Read the model definition and answer for the solid it produces. Units are mm, in the model's axes. Coordinates: 2 decimals unless noted, no trailing zeros. Loops run counter-clockwise (first coordinate to the right, second up) from the corner with the lowest first, then second, coordinate; pieces in that order, holes last. Notation, with made-up numbers: (68, -16.75) -> (76, -16.75) arc R23 ccw to (76, 14.25) -> close; hole circle Ø6 at (-24.5, 16.25). An arc over 180 degrees is marked (long way). Answer in a Markdown table with one row per item.
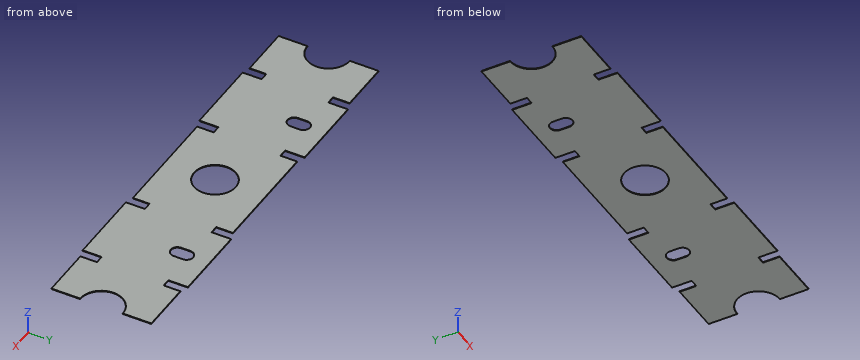
```python
from build123d import *

# Parameters (mm, degrees)
SKETCH_1_R      = 5
EXTRUDE_1_DEPTH = 0.15


with BuildPart() as part:
    # Эскиз1 → Бобышка-Вытянуть1 (new body)
    with BuildSketch(Plane(origin=(0, 0, 0), x_dir=(-1, 0, 0), z_dir=(0, 0, -1))):
        with BuildLine():
            Line((-94.25, 76.699996948), (-94.25, 72))
            Line((-94.25, 72), (-96.25, 72))
            Line((-96.25, 72), (-96.25, 76))
            Line((-96.25, 76), (-108.650001526, 76))
            Line((-108.650001526, 76), (-108.650001526, 69.126998901))
            ThreePointArc((-108.650001526, 69.126998901), (-103.523002625, 64), (-108.650001526, 58.873001099))
            Line((-108.650001526, 58.873001099), (-108.650001526, 52))
            Line((-108.650001526, 52), (-96.25, 52))
            Line((-96.25, 52), (-96.25, 56))
            Line((-96.25, 56), (-94.25, 56))
            Line((-94.25, 56), (-94.25, 51.424999237))
            Line((-94.25, 51.424999237), (-75.75, 51.424999237))
            Line((-75.75, 51.424999237), (-75.75, 56))
            Line((-75.75, 56), (-73.75, 56))
            Line((-73.75, 56), (-73.75, 52))
            Line((-73.75, 52), (-46.25, 52))
            Line((-46.25, 52), (-46.25, 56))
            Line((-46.25, 56), (-44.25, 56))
            Line((-44.25, 56), (-44.25, 51.424999237))
            Line((-44.25, 51.424999237), (-25.75, 51.424999237))
            Line((-25.75, 51.424999237), (-25.75, 56))
            Line((-25.75, 56), (-23.75, 56))
            Line((-23.75, 56), (-23.75, 52))
            Line((-23.75, 52), (-11.350000381, 52))
            Line((-11.350000381, 52), (-11.350000381, 58.909999847))
            ThreePointArc((-11.350000381, 58.909999847), (-16.439998627, 63.999998093), (-11.350000381, 69.089996338))
            Line((-11.350000381, 69.089996338), (-11.350000381, 76))
            Line((-11.350000381, 76), (-23.75, 76))
            Line((-23.75, 76), (-23.75, 72))
            Line((-23.75, 72), (-25.75, 72))
            Line((-25.75, 72), (-25.75, 76.699996948))
            Line((-25.75, 76.699996948), (-44.25, 76.699996948))
            Line((-44.25, 76.699996948), (-44.25, 72))
            Line((-44.25, 72), (-46.25, 72))
            Line((-46.25, 72), (-46.25, 76))
            Line((-46.25, 76), (-73.75, 76))
            Line((-73.75, 76), (-73.75, 72))
            Line((-73.75, 72), (-75.75, 72))
            Line((-75.75, 72), (-75.75, 76.699996948))
            Line((-75.75, 76.699996948), (-94.25, 76.699996948))
        make_face()
        with Locations((-60.017142334, 64)):
            Circle(SKETCH_1_R, mode=Mode.SUBTRACT)
        with BuildLine():
            Line((-33.400001526, 68.999998474), (-33.400001526, 71.199998474))
            ThreePointArc((-33.400001526, 71.199998474), (-35, 72.799996948), (-36.599998474, 71.199998474))
            Line((-36.599998474, 71.199998474), (-36.599998474, 68.999998474))
            ThreePointArc((-36.599998474, 68.999998474), (-35, 67.4), (-33.400001526, 68.999998474))
        make_face(mode=Mode.SUBTRACT)
        with BuildLine():
            Line((-83.400001526, 71.199998474), (-83.400001526, 68.999998474))
            ThreePointArc((-83.400001526, 68.999998474), (-85, 67.4), (-86.599998474, 68.999998474))
            Line((-86.599998474, 68.999998474), (-86.599998474, 71.199998474))
            ThreePointArc((-86.599998474, 71.199998474), (-85, 72.799996948), (-83.400001526, 71.199998474))
        make_face(mode=Mode.SUBTRACT)
    extrude(amount=-EXTRUDE_1_DEPTH)


solid = part.part
```
1. A cutting plane is placed at C-C on z = 0.05. Count the separate pieces of the cut face and the enclosed holes in it, and give its area (3 significant figures).
A:
| item | result |
|---|---|
| separate pieces | 1 |
| enclosed holes | 3 |
| area | 2,130 mm2 |
2. A cutting plane is placed at B-B on x = 35. Give the vertices of the cut face in (y, z) (3 decimals).
A:
| item | result |
|---|---|
| outline | (51.425, 0) -> (67.4, 0) -> (67.4, 0.15) -> (51.425, 0.15) -> close; (72.8, 0) -> (76.7, 0) -> (76.7, 0.15) -> (72.8, 0.15) -> close |
3. Find the intervals of material crossed by probe 1 along X at (y, z) = (70.5, 0.1); probe 2 along X at (y, z) = (53.25, 0.1); probe 3 along Y at (x, z) = (34, 0.1) (3 decimals), in increasing order.
A:
| item | result |
|---|---|
| probe 1 | x = 11.35 to 33.4, 36.6 to 83.4, 86.6 to 108.65 |
| probe 2 | x = 11.35 to 23.75, 25.75 to 44.25, 46.25 to 73.75, 75.75 to 94.25, 96.25 to 108.65 |
| probe 3 | y = 51.425 to 67.751, 72.449 to 76.7 |
4. A cutting plane is placed at D-D on x = 66.5. Give the vertices of the cut face in (y, z), and give its area (3 significant figures).
A:
| item | result |
|---|---|
| outline | (52, 0) -> (76, 0) -> (76, 0.15) -> (52, 0.15) -> close |
| area | 3.60 mm2 |
5. A cutting plane is placed at A-A on y = 64. Give the vertices of the cut face in (x, z), and give its area (3 significant figures).
A:
| item | result |
|---|---|
| outline | (16.44, 0) -> (55.02, 0) -> (55.02, 0.15) -> (16.44, 0.15) -> close; (65.02, 0) -> (103.52, 0) -> (103.52, 0.15) -> (65.02, 0.15) -> close |
| area | 11.6 mm2 |
